Autodesk Inventor part; units mm, degrees
ref_plane "Work Plane1" through (0, 0, -15) normal (0, 0, 1) x (1, 0, 0)
ref_plane "YZ Plane" through (0, 0, 0) normal (1, 0, 0) x (0, 1, 0)
ref_plane "XZ Plane" through (0, 0, 0) normal (0, 1, 0) x (-1, 0, 0)
sketch "Sketch1" plane through (0, 0, 0) normal (0, 0, 1) x (1, 0, 0)
  line L0 (0, 0) -> (25, 0)
  line L1 (25, 0) -> (25, 40)
  line L2 (25, 40) -> (0, 40)
  line L3 (0, 40) -> (0, 0)
  dimension "d1" = 25
  dimension "d2" = 40
  dimension "d3" = 25
extrude "Extrusion1" add sketch "Sketch1" against normal blind 30
sketch "Sketch2" plane through (25, 0, 0) normal (1, 0, 0) x (0, 0, -1)
  line L0 (0, 0) -> (30, 0)
  circle A0 centre (15, 6.56) radius 2.46
extrude "Extrusion2" cut sketch "Sketch2" against normal blind 30
sketch "Sketch3" plane through (0, 0, 0) normal (-1, 0, 0) x (0, 0, 1)
  line L0 (0, 0) -> (-30, 0)
  line L1 (-25.05, 0) -> (-4.95, 0)
  line L2 (-4.95, 0) -> (-4.95, 33.12)
  line L3 (-4.95, 33.12) -> (-25.05, 33.12)
  line L4 (-25.05, 33.12) -> (-25.05, 0)
  dimension "d11" = 20.1
extrude "Extrusion3" cut sketch "Sketch3" against normal blind 20
sketch "Sketch4" plane through (0, 0, 0) normal (0, -1, 0) x (1, 0, 0)
  line L0 (20, -4.95) -> (20, -25.05)
  line L1 (20, -15) -> (25, -15)
  line L2 (25, 0) -> (25, -30)
  line L3 (20, -8.025) -> (25, -8.025)
  line L4 (25, -8.025) -> (25, -21.975)
  line L5 (25, -21.975) -> (20, -21.975)
  line L6 (20, -21.975) -> (20, -8.025)
  line L7 (20, -8.025) -> (25, -21.975) construction
  line L8 (25, -8.025) -> (20, -21.975) construction
  line L9 (25, -12.54) -> (25, -17.46)
  point P0 (0, 0)
  point P1 (22.5, -15)
  dimension "d14" = 13.95
extrude "Extrusion4" add sketch "Sketch4" along normal blind 15
sketch "Sketch5" plane through (20, 0, 0) normal (-1, 0, 0) x (0, 0, 1)
  circle A0 centre (-15, 6.56) radius 2.46
  circle A1 centre (-15, 6.56) radius 4.7025
  circle A2 centre (-15, 6.56) radius 2.46
  circle A3 centre (-15, 6.56) radius 2.46
  point P0 (0, 0)
  dimension "d17" = 9.405
extrude "Extrusion5" cut sketch "Sketch5" against normal blind 2.1
sketch "Sketch6" plane through (25, 0, 0) normal (1, 0, 0) x (0, 0, -1)
  circle A0 centre (15, 6.56) radius 4.7025
  line L0 (15, 6.56) -> (15, 23.56)
  circle A1 centre (15, 23.56) radius 2.46
  point P0 (0, 0)
  dimension "d20" = 17
  dimension "d21" = 4.92
extrude "Extrusion6" cut sketch "Sketch6" against normal blind 10 contours A1
sketch "Sketch7" plane through (20, 0, 0) normal (-1, 0, 0) x (0, 0, 1)
  circle A0 centre (-15, 23.56) radius 2.46
  circle A1 centre (-15, 23.56) radius 4.7025
  point P0 (0, 0)
  dimension "d24" = 9.405
extrude "Extrusion7" cut sketch "Sketch7" against normal blind 2.1
sketch "Sketch9" plane through (25, 0, 0) normal (1, 0, 0) x (0, 0, -1)
  circle A0 centre (15, 6.56) radius 2.46
  circle A1 centre (15, 6.56) radius 2.46
  circle A2 centre (15, 23.56) radius 2.46
  circle A3 centre (15, 23.56) radius 2.46
  line L0 (30, 40) -> (30, 0)
  line L1 (30, 0) -> (30, 40)
  line L2 (30, 40) -> (0, 40)
  line L3 (0, 40) -> (0, 0)
  line L4 (0, 0) -> (8.025, 0)
  line L5 (21.975, 0) -> (21.975, -15)
  line L6 (21.975, -15) -> (8.025, -15)
  line L7 (8.025, -15) -> (8.025, 0)
  line L8 (0, 0) -> (8.025, 0)
  line L9 (21.975, 0) -> (30, 0)
extrude "Extrusion8" add sketch "Sketch9" along normal blind 5
sketch "Sketch10" plane through (0, 40, 0) normal (0, 1, 0) x (1, 0, 0)
  line L0 (0, 30) -> (30, 30)
  line L1 (30, 0) -> (0, 0)
  line L2 (0, 30) -> (30, 30)
  line L3 (30, 30) -> (30, 0)
  line L4 (30, 0) -> (0, 0)
  line L5 (0, 0) -> (0, 30)
extrude "Extrusion9" add sketch "Sketch10" along normal blind 30
sketch "Sketch12" plane through (30, 0, 0) normal (1, 0, 0) x (0, 0, -1)
  circle A0 centre (15, 6.56) radius 2.46
  line L0 (15, 6.56) -> (15, 15.06)
  circle A1 centre (15, 15.06) radius 2.525
  point P0 (0, 0)
  dimension "d31" = 8.5
  dimension "d33" = 5.05
extrude "Extrusion10" cut sketch "Sketch12" against normal blind 30 contours A1
sketch "Sketch14" plane through (0, 0, 0) normal (0, 0, 1) x (1, 0, 0)
  line L0 (30, 70) -> (0, 70)
  line L1 (0, 70) -> (0, 85)
  line L2 (30, 0) -> (30, 70)
  line L3 (30, 113) -> (30, 70)
  line L4 (30, 105) -> (30, 100)
  line L5 (-12, 128) -> (15, 128)
  line L6 (-8, 126) -> (-12, 128)
  line L7 (-8, 126) -> (-4, 114)
  line L8 (-8, 102) -> (-12, 100)
  line L9 (-8, 102) -> (-4, 114)
  line L10 (30, 113) -> (15, 128)
  line L11 (0, 100) -> (-12, 100)
  line L12 (0, 100) -> (0, 85)
  point P0 (0, 0)
  dimension "d69" = 28
  dimension "d74" = 12
extrude "Extrusion12" add sketch "Sketch14" against normal blind 30
sketch "Sketch15" plane through (0, 0, -25.05) normal (-1, 0, 0) x (0, 0, 1)
  line L0 (0, 33.12) -> (20.1, 33.12)
  line L1 (20.1, 33.12) -> (20.1, 0)
  line L2 (0, 33.12) -> (20.1, 33.12)
  line L3 (20.1, 33.12) -> (20.1, 31.1)
  line L4 (20.1, 31.1) -> (0, 31.1)
  line L5 (0, 31.1) -> (0, 33.12)
  point P0 (25.05, 0)
  dimension "d57" = 2.02
extrude "Extrusion13" add sketch "Sketch15" against normal blind 20
sketch "Sketch21" plane through (0, 0, 0) normal (0, 0, 1) x (1, 0, 0)
  line L0 (0, 100) -> (-12, 100)
  line L1 (0, 100) -> (-12, 100)
  line L2 (-12, 100) -> (-8, 102)
  line L3 (-12, 100) -> (-8, 102)
  line L4 (-8, 102) -> (-4, 114)
  line L5 (-8, 102) -> (-4, 114)
  line L6 (-4, 114) -> (-8, 126)
  line L7 (-4, 114) -> (-8, 126)
  line L8 (-8, 126) -> (-12, 128)
  line L9 (-8, 126) -> (-12, 128)
  line L10 (-12, 128) -> (15, 128)
  line L11 (-12, 128) -> (15, 128)
  line L12 (15, 128) -> (30, 113)
  line L13 (15, 128) -> (30, 113)
  line L14 (30, 113) -> (30, 93)
  line L15 (30, 0) -> (30, 113)
  line L16 (30, 93) -> (0, 93)
  line L17 (0, 93) -> (0, 100)
  point P0 (0, 0)
  dimension "d75" = 20
  dimension "d76" = 30
extrude "Extrusion14" add sketch "Sketch21" along normal blind 30
ref_plane "Work Plane1" through (0, 0, -15) normal (0, 0, 1) x (1, 0, 0)
mirror "Mirror1" about plane through (0, 0, -15) normal (0, 0, 1) of "Extrusion14"
properties part number "rec_b_24mm_x_90mm"
The listing builds one solid part. Answer for the finished solid, in the listing's coordinates (mm). A direction names the side the tool comes from. Coordinates: 2 decimals unless noted, no trailing zeros. Order: outer loops, then holes, each group sorted by start corner. A loop starts at its lowest first (then second) coordinate and runs counter-clockwise, first axis right, second up. Notation, with made-up numbers: M 55.25,69 L 111.25,69 A25 cw 111.25,88 Z; hole C 47,-37.5 d8. An arc over 180 degrees is marked long. Use CSV: the item, a comma, the result in double quotes.
Q1. Section B-B (x = 25.5) is taken. Determine the outline of the cut face in (y, z) (3 decimals).
Here are the results:
outline,"M -15,-21.975 L 0,-21.975 L 0,-30 L 93,-30 L 93,-60 L 117.5,-60 L 117.5,30 L 93,30 L 93,0 L 0,0 L 0,-8.025 L -15,-8.025 Z; hole C 6.56,-15 d4.92; hole C 15.06,-15 d5.05; hole C 23.56,-15 d4.92"
Q2. Straight lines are drawn through the part: L1, parallel to Y at x = 25, z = -15 (3 decimals); L2, parallel to Z at x = 23.25, y = 15.06 (3 decimals); L3, parallel to Z at x = 7, y = 8. For each, find the intervals that lie inside material, in ascending order.
Here are the results:
L1,"-15 to 4.1, 9.02 to 12.535, 17.585 to 21.1, 26.02 to 118"
L2,"-30 to -17.525, -12.475 to 0"
L3,"-30 to -25.05, -4.95 to 0"
Q3. A tool of negligible diameter and unlimited length cuts with its end or side. For faces 1 (the flat face through (0, 65, -15)), 2 (the flat face through (15, 93, -45)), 3 (the flat face through (-10, 127, -14)), from which of +Z, -Z, +X, -X, +Y, -Y can it reach the whole face along a straight path? Write none if from no direction.
Here are the results:
face 1,"+Z, -Z, -X, -Y"
face 2,"-Z, +X, -X, -Y"
face 3,"+Z, -Z, -X"
Q4. Section D-D (z = 3) is taken. Determine the outline of the cut face in (x, y).
Here are the results:
outline,"M -12,100 L 0,100 L 0,93 L 30,93 L 30,113 L 15,128 L -12,128 L -8,126 L -4,114 L -8,102 Z"
Q5. Determine the mould class of faces 4 (the flat face through (10, 16, -25.05)), 5 (the flat face through (-6, 120, -14)), 6 (the flat face through (15, 47, 0)) for opening direction Z: pulls with the +Z half, pulls with the -Z half, needs draft (parallel to the pull), parting line crosses it, or undercut.
Here are the results:
face 4,"undercut"
face 5,"needs draft"
face 6,"pulls with the +Z half"
Q6. Given pin 1 Ø4 at (x, z) = (0.5, -21.5) entering from -Y; pin 2 Ø10 at (x, y) = (10, 22.5) entering from +Z; pin 3 Ø5 at (x, y) = (25, -10.5) entering from +Z (3 decimals); pin 4 Ø4.5 at (y, z) = (23.56, -15) entering from -X, each flat-ended and moving along its own axis, determine where each tip first touches the part or whether it passes through.
Here are the results:
pin 1,"y = 31.1"
pin 2,"z = 0"
pin 3,"z = -8.025"
pin 4,"through"
Q7. Section C-C (y = 6.56) is taken. Determine the outline of the cut face in (x, z).
Here are the results:
outline,"M 0,-30 L 30,-30 L 30,-17.46 L 22.1,-17.46 L 22.1,-19.7 L 20,-19.7 L 20,-25.05 L 0,-25.05 Z; M 0,-4.95 L 20,-4.95 L 20,-10.3 L 22.1,-10.3 L 22.1,-12.54 L 30,-12.54 L 30,0 L 0,0 Z"
Q8. Section A-A (z = -15) is taken. Give the number of separate pieces and of enclosed holes in the cut face, then the cut area to 3 significant figures.
Here are the results:
separate pieces,"4"
enclosed holes,"0"
area,"3,270 mm2"
